Here's the drawing with two shaded views (mm, measured from the low corner). I have some questions. Coordinates: 2 decimals unless noted, no trailing zeros. Write each loop counter-clockwise with the first axis right and the second up, starting at its lowest first coordinate (ties: lowest second). Pieces come first, ordered by that corner, then holes. Notation, with made-up numbers: (-19.5, 24) -> (-12.5, 24) arc R13 ccw to (-12.5, 46) -> close; hole circle Ø7 at (-21, 26.25). An arc over 180 degrees is marked (long way). Use a Markdown table: item, result. Add a question column.
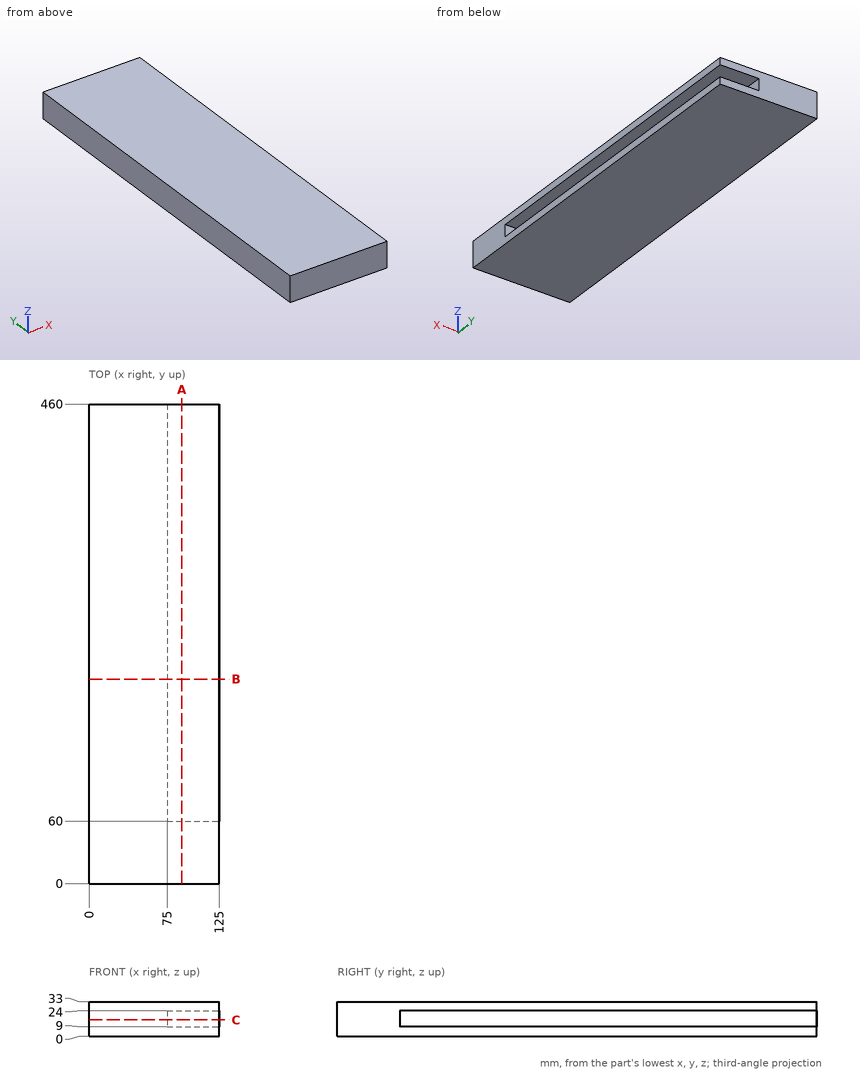
Q1. Suppose I cut it at C-C, the plane z = 15.5. Write out the boundary of the cut face in (x, y).
Q2. Please list where these lines run through material, in increasing order: line 1 (Z direction, x = 108, y = 410.5); line 2 (Y direction, x = 78, z = 10); line 3 (X direction, y = 441, z = 20).
Q3. Suppose I cut it at B-B, the plane y = 196. Write out the boundary of the cut face in (x, z).
Q4. Will this pin go through, and if not, where does the flat tip stop? pin 1 (2 mm diameter, centred on y = 264.5, z = 18, fed in from +X).
Q5. Suppose I cut it at A-A, the plane x = 89. Write out the boundary of the cut face in (y, z).
Answer key:
| question | item | result |
|---|---|---|
| 1 | outline | (0, 0) -> (125, 0) -> (125, 60) -> (75, 60) -> (75, 460) -> (0, 460) -> close |
| 2 | line 1 | z = 0 to 9, 24 to 33 |
| 2 | line 2 | y = 0 to 60 |
| 2 | line 3 | x = 0 to 75 |
| 3 | outline | (0, 0) -> (125, 0) -> (125, 9) -> (75, 9) -> (75, 24) -> (125, 24) -> (125, 33) -> (0, 33) -> close |
| 4 | pin 1 | stops at x = 75 |
| 5 | outline | (0, 0) -> (460, 0) -> (460, 9) -> (60, 9) -> (60, 24) -> (460, 24) -> (460, 33) -> (0, 33) -> close |
